```python
from build123d import *

# Parameters (mm, degrees)
SKETCH_R     = 1.5
SKETCH_R_2   = 11
PAD_DEPTH    = 3
SKETCH003_W  = 60
SKETCH003_H  = 3
PAD001_DEPTH = 22
SKETCH002_R  = 1.5
POCKET_DEPTH = 3
FILLET_R     = 3


with BuildPart() as part:
    # Sketch → Pad (new body)
    with BuildSketch(Plane.XZ):
        with BuildLine():
            ThreePointArc((16.910328, 32.50272), (0, 43.5), (-16.910328, 32.50272))
            Line((-30, 3), (-16.910328, 32.50272))
            Line((-30, 0), (-30, 3))
            Line((-30, 0), (30, 0))
            Line((30, 0), (30, 3))
            Line((30, 3), (16.910328, 32.50272))
        make_face()
        with Locations((10, 15)):
            Circle(SKETCH_R, mode=Mode.SUBTRACT)
        with Locations((10, 35)):
            Circle(SKETCH_R, mode=Mode.SUBTRACT)
        with Locations((-10, 35)):
            Circle(SKETCH_R, mode=Mode.SUBTRACT)
        with Locations((-10, 15)):
            Circle(SKETCH_R, mode=Mode.SUBTRACT)
        with Locations((0, 25)):
            Circle(SKETCH_R_2, mode=Mode.SUBTRACT)
    extrude(amount=PAD_DEPTH)

    # Sketch003 (on Face13 of Pad) → Pad001 (join)
    with BuildSketch(Plane.XZ.offset(3)):
        with Locations((0, 1.5)):
            Rectangle(SKETCH003_W, SKETCH003_H)
    extrude(amount=PAD001_DEPTH)

    # Sketch002 → Pocket (cut)
    with BuildSketch(Plane(origin=(0, 0, 3), x_dir=(-1, 0, 0), z_dir=(0, 0, 1))):
        with Locations((23, 19)):
            Circle(SKETCH002_R)
        with Locations((23, 9)):
            Circle(SKETCH002_R)
        with Locations((-23, 19)):
            Circle(SKETCH002_R)
        with Locations((-23, 9)):
            Circle(SKETCH002_R)
        with Locations((0, 14)):
            Circle(SKETCH002_R)
    extrude(amount=-POCKET_DEPTH, mode=Mode.SUBTRACT)

    # Fillet
    fillet_edges = [part.edges().sort_by_distance(p)[0] for p in [
        (30, -25, 1.5),
        (-30, -25, 1.5),
    ]]
    fillet(fillet_edges, radius=FILLET_R)


solid = part.part
```
Source: CAD feature listing. Evaluate the final solid. Frame: model axes, mm. A direction names the side the tool comes from. Give positions to 0.01 mm unless a question says otherwise; leave off trailing zeros. Loops run counter-clockwise (first coordinate to the right, second up) from the corner with the lowest first, then second, coordinate; pieces in that order, holes last. Notation, with made-up numbers: (60.25, 45) - (110.25, 45) arc R35 ccw to (110.25, 81) - close; hole circle Ø1 at (40, 16). An arc over 180 degrees is marked (long way). Use CSV: the item, a comma, the result in double quotes. Start each with the question number.
1. Section B-B (y = -14). Output: boundary loops of the cut face in (x, z), then the cut area to 3 significant figures.
2. Section D-D (x = 4). Output: boundary loops of the cut face in (y, z).
3. Pin query (flat end, axial travel): pin 1 (3 mm diameter, centred on y = -4, z = 23.5, fed in from -X); pin 2 (5 mm diameter, centred on x = -23, y = -9, fed in from +Z); pin 3 (5 mm diameter, centred on x = -10, z = 35, fed in from -Y); pin 4 (3.5 mm diameter, centred on x = -23, y = -19, fed in from -Z). Return the tip coordinate at first contact, or that it passes through.
4. Section C-C (z = 35). Output: boundary loops of the cut face in (x, y), then the cut area to 3 significant figures.
5. Draft query along Z for faces 3 (the flat face through (0, -12, 0)), 4 (the cylindrical face through (29.1, -24.14, 1.52)), 5 (the cylindrical face through (-2.38, -1.48, 14.26)). Return one class per face: +Z half, -Z half, draft (parallel to the pull), parting line (faces both ways), or undercut.
6. Section A-A (y = -9). Output: boundary loops of the cut face in (x, z).
7. Ray query, L1, parallel to Y at x = -23, z = 1.7; L2, parallel to Z at x = 0, y = -1.05; L3, parallel to Z at x = -10, y = -1.8. Return the intervals inside material, ascending.
8. Reachability of faces 1 (the flat face through (0, -16, 3)), 2 (the cylindrical face through (-29.14, -24.1, 1.52)) from +Z, -Z, +X, -X, +Y, -Y: full face, straight path, thin tool, end or side. Return the list, or none.
Response:
1,outline,"(-30, 0) - (-1.5, 0) - (-1.5, 3) - (-30, 3) - close; (1.5, 0) - (30, 0) - (30, 3) - (1.5, 3) - close"
1,area,"171 mm²"
2,outline,"(-25, 0) - (0, 0) - (0, 14.75) - (-3, 14.75) - (-3, 3) - (-25, 3) - close; (-3, 35.25) - (0, 35.25) - (0, 43.06) - (-3, 43.06) - close"
3,pin 1,"x = -21.4"
3,pin 2,"z = 3"
3,pin 3,"y = -3"
3,pin 4,"z = 0"
4,outline,"(-15.56, -3) - (-11.5, -3) - (-11.5, 0) - (-15.56, 0) - close; (-8.5, -3) - (-4.58, -3) - (-4.58, 0) - (-8.5, 0) - close; (4.58, -3) - (8.5, -3) - (8.5, 0) - (4.58, 0) - close; (11.5, -3) - (15.56, -3) - (15.56, 0) - (11.5, 0) - close"
4,area,"47.9 mm²"
5,face 3,"-Z half"
5,face 4,"draft"
5,face 5,"undercut"
6,outline,"(-30, 0) - (-24.5, 0) - (-24.5, 3) - (-30, 3) - close; (-21.5, 0) - (21.5, 0) - (21.5, 3) - (-21.5, 3) - close; (24.5, 0) - (30, 0) - (30, 3) - (24.5, 3) - close"
7,L1,"-25 to -20.5, -17.5 to -10.5, -7.5 to 0"
7,L2,"0 to 14, 36 to 43.5"
7,L3,"0 to 13.5, 16.5 to 20.42, 29.58 to 33.5, 36.5 to 40.56"
8,face 1,"+Z, +X, -X, -Y"
8,face 2,"+Z, -Z, -X, -Y"
